from build123d import *

# Parameters (mm, degrees)
SKETCH2_R           = 2.5
BOSS_EXTRUDE1_DEPTH = 5
SKETCH3_R           = 5
BOSS_EXTRUDE2_DEPTH = 15
SKETCH4_R           = 0.75
CUT_EXTRUDE1_DEPTH  = 15
SKETCH5_R           = 1.25
CUT_EXTRUDE2_DEPTH  = 1
CUT_EXTRUDE3_DEPTH  = 1


with BuildPart() as part:
    # Sketch2 → Boss-Extrude1 (new body)
    with BuildSketch(Plane(origin=(0, 0, 0), x_dir=(1, 0, 0), z_dir=(0, 1, 0))):
        with Locations(Location((0, 0, 0), (0, 0, 270))):
            Circle(SKETCH2_R)
    extrude(amount=BOSS_EXTRUDE1_DEPTH)

    # Sketch3 → Boss-Extrude2 (add)
    with BuildSketch(Plane(origin=(0, 5, 0), x_dir=(1, 0, 0), z_dir=(0, 1, 0))):
        with Locations(Location((0, 0, 0), (0, 0, 270))):
            Circle(SKETCH3_R)
    extrude(amount=BOSS_EXTRUDE2_DEPTH)

    # Sketch4 → Cut-Extrude1 (cut)
    with BuildSketch(Plane(origin=(0, 20, 0), x_dir=(1, 0, 0), z_dir=(0, 1, 0))):
        with Locations((0, 5)):
            Circle(SKETCH4_R)
        with Locations((3.909157412, 3.117449009)):
            Circle(SKETCH4_R)
        with Locations((4.874639561, -1.11260467)):
            Circle(SKETCH4_R)
        with Locations((2.169418696, -4.50484434)):
            Circle(SKETCH4_R)
        with Locations((-2.169418696, -4.50484434)):
            Circle(SKETCH4_R)
        with Locations((-4.874639561, -1.11260467)):
            Circle(SKETCH4_R)
        with Locations((-3.909157412, 3.117449009)):
            Circle(SKETCH4_R)
    extrude(amount=-CUT_EXTRUDE1_DEPTH, mode=Mode.SUBTRACT)

    # Sketch5 → Cut-Extrude2 (cut)
    with BuildSketch(Plane.XZ):
        with Locations(Location((0, 0, 0), (0, 0, 270))):
            Circle(SKETCH5_R)
    extrude(amount=-CUT_EXTRUDE2_DEPTH, mode=Mode.SUBTRACT)

    # Sketch6 → Cut-Extrude3 (cut)
    with BuildSketch(Plane.XZ):
        with BuildLine():
            Line((-0.5, 2.449489743), (-0.5, 1.145643924))
            ThreePointArc((-0.5, 1.145643924), (0, 1.25), (0.5, 1.145643924))
            Line((0.5, 1.145643924), (0.5, 2.449489743))
            ThreePointArc((0.5, 2.449489743), (0, 2.5), (-0.5, 2.449489743))
        make_face()
    extrude(amount=-CUT_EXTRUDE3_DEPTH, mode=Mode.SUBTRACT)


solid = part.part
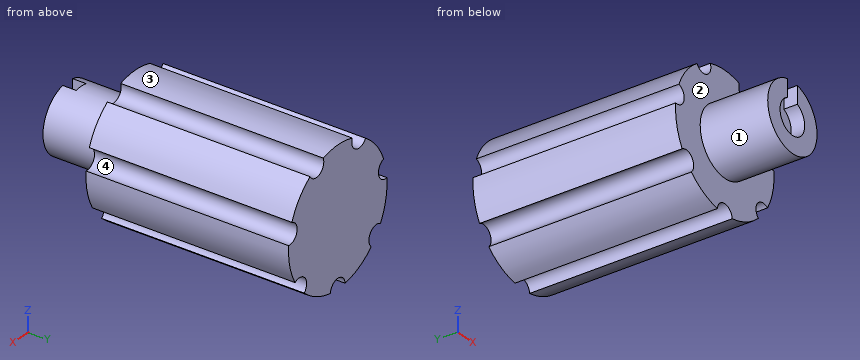
Verification items for the finished model (mm, model axes). Face numbers are marked on the shaded views. Round coordinates to 2 decimals unless told otherwise and drop trailing zeros. Write each loop counter-clockwise with the first axis right and the second up, starting at its lowest first coordinate (ties: lowest second). Pieces come first, ordered by that corner, then holes.
(1) Section check D-D (x = -2). Enter the section's corners in (y, z), plus the area to 3 significant figures.
Returned:
outline: (0, -1.5) - (5, -1.5) - (5, -4.58) - (20, -4.58) - (20, 3.77) - (5, 3.77) - (5, 1.5) - (0, 1.5) - close
area: 140 mm2
(2) Section check A-A (x = 0). Enter the section's corners in (y, z), plus the area to 3 significant figures.
Returned:
outline: (0, -2.5) - (5, -2.5) - (5, -4.25) - (20, -4.25) - (20, 5) - (5, 5) - (5, 2.5) - (1, 2.5) - (1, -1.25) - (0, -1.25) - close
area: 160 mm2
(3) Mould release check, pull along Z, two halves, no side actions. Record for the marked faces 1, 2, 3 and 4: pulls with the +Z half, pulls with the -Z half, needs draft (parallel to the pull), parting line crosses it, or undercut.
Returned:
face 1: parting line crosses it
face 2: needs draft
face 3: pulls with the +Z half
face 4: undercut
(4) Depth check by flat-ended pin: pin 1 Ø1.2 at (x, z) = (0, 0.5) entering from -Y; pin 2 Ø0.5 at (y, z) = (0.5, 2) entering from -X; pin 3 Ø3 at (x, y) = (1.5, 14) entering from +Z; pin 4 Ø1.1 at (y, z) = (0.5, 2) entering from +X. Enter the tip coordinate at first touch or a pass-through.
Returned:
pin 1: stops at y = 1
pin 2: stops at x = -1.79
pin 3: stops at z = 5
pin 4: stops at x = 2.04
(5) Section check C-C (y = 8.75). Enter the section's corners in (x, z), plus the area to 3 significant figures.
Returned:
outline: (-4.99, 0.37) arc R5 ccw to (-4.33, -2.5) arc R0.75 cw to (-3.4, -3.67) arc R5 ccw to (-0.75, -4.94) arc R0.75 cw to (0.75, -4.94) arc R5 ccw to (3.4, -3.67) arc R0.75 cw to (4.33, -2.5) arc R5 ccw to (4.99, 0.37) arc R0.75 cw to (4.65, 1.83) arc R5 ccw to (2.82, 4.13) arc R0.75 cw to (1.47, 4.78) arc R5 ccw to (-1.47, 4.78) arc R0.75 cw to (-2.82, 4.13) arc R5 ccw to (-4.65, 1.83) arc R0.75 cw to start
area: 72.6 mm2
(6) Material ranges on line 1 (X direction, y = 0.4, z = 0); line 2 (X direction, y = 14.25, z = 4.5); line 3 (Z direction, x = 0, y = 0.2), recorded low to high.
Returned:
line 1: x = -2.5 to -1.25, 1.25 to 2.5
line 2: x = -1.42 to 1.42
line 3: z = -2.5 to -1.25
(7) Section check B-B (z = 0). Enter the section's corners in (x, y), plus the area to 4 significant figures.
Returned:
outline: (-5, 5) - (-2.5, 5) - (-2.5, 0) - (-1.25, 0) - (-1.25, 1) - (1.25, 1) - (1.25, 0) - (2.5, 0) - (2.5, 5) - (5, 5) - (5, 20) - (-5, 20) - close
area: 172.5 mm2
